Here's how the part is built. I have some questions about the finished solid (model axes, mm). A direction names the side the tool comes from. Round coordinates to 2 decimals unless told otherwise and drop trailing zeros. One line per item, written item: value. Start each with the question number.
```python
from build123d import *

# Parameters (mm, degrees)
BOSS_EXTRUDE1_DEPTH = 5
SKETCH4_W           = 22
SKETCH4_H           = 25.575781223
CUT_EXTRUDE1_DEPTH  = 5
CUT_EXTRUDE2_DEPTH  = 5
SKETCH10_W          = 47.253020793
SKETCH10_H          = 79.148030785
CUT_EXTRUDE3_DEPTH  = 5
MIRROR8_DEPTH       = 5
SKETCH11_R          = 10.33
CUT_EXTRUDE4_DEPTH  = 5
FILLET5_R           = 2


# Read off the part's stored shape, not the designer's step: Mirror8
with BuildPart() as part:
    # Sketch3 → Boss-Extrude1 (new body)
    with BuildSketch(Plane(origin=(0, 0, 0), x_dir=(1, 0, 0), z_dir=(0, 1, 0))):
        Polygon((35, 0), (24.748737342, 24.748737342), (0, 35), (-24.748737342, 24.748737342), (-35, 0), (-24.748737342, -24.748737342), (0, -35), (24.748737342, -24.748737342), align=None)
    extrude(amount=BOSS_EXTRUDE1_DEPTH)

    # Sketch4 → Cut-Extrude1 (cut)
    with BuildSketch(Plane(origin=(0, 5, 0), x_dir=(1, 0, 0), z_dir=(0, 1, 0))):
        with Locations((-11.044164743, -6.541737694)):
            Rectangle(SKETCH4_W, SKETCH4_H)
    extrude(amount=-CUT_EXTRUDE1_DEPTH, mode=Mode.SUBTRACT)

    # Sketch4<6> → Cut-Extrude2 (cut)
    with BuildSketch(Plane(origin=(0, 5, 0), x_dir=(1, 0, 0), z_dir=(0, 1, 0))):
        with BuildLine():
            ThreePointArc((-22.044164743, 6.246152918), (-11.044164743, 10.694704781), (-0.044164743, 6.246152918))
            Line((-0.044164743, 6.246152918), (-22.044164743, 6.246152918))
        make_face()
        with BuildLine():
            Line((-22.044164743, -19.329628305), (-0.044164743, -19.329628305))
            ThreePointArc((-0.044164743, -19.329628305), (-11.044164743, -23.778180168), (-22.044164743, -19.329628305))
        make_face()
    extrude(amount=-CUT_EXTRUDE2_DEPTH, mode=Mode.SUBTRACT)

    # Sketch10 → Cut-Extrude3 (cut)
    with BuildSketch(Plane(origin=(0, 5, 0), x_dir=(1, 0, 0), z_dir=(0, 1, 0))):
        with Locations((23.626510397, -1.493894903)):
            Rectangle(SKETCH10_W, SKETCH10_H)
    extrude(amount=-CUT_EXTRUDE3_DEPTH, mode=Mode.SUBTRACT)

    # Mirror8 outline → Mirror8 (add)
    with BuildSketch(Plane(origin=(0, 0, 0), x_dir=(1, 0, 0), z_dir=(0, 1, 0))):
        Polygon((24.748737342, 24.748737342), (0, 35), (0, -35), (24.748737342, -24.748737342), (35, 0), align=None)
        with BuildLine():
            ThreePointArc((0.044164743, 6.246152918), (11.044164743, 10.694704781), (22.044164743, 6.246152918))
            Line((22.044164743, 6.246152918), (22.044164743, -19.329628305))
            ThreePointArc((22.044164743, -19.329628305), (11.044164743, -23.778180168), (0.044164743, -19.329628305))
            Line((0.044164743, -19.329628305), (0.044164743, 6.246152918))
        make_face(mode=Mode.SUBTRACT)
    extrude(amount=MIRROR8_DEPTH)

    # Sketch11 → Cut-Extrude4 (cut)
    with BuildSketch(Plane(origin=(0, 5, 0), x_dir=(1, 0, 0), z_dir=(0, 1, 0))):
        with Locations(Location((0, 18.670604022, 0), (0, 0, 270))):
            Circle(SKETCH11_R)
    extrude(amount=-CUT_EXTRUDE4_DEPTH, mode=Mode.SUBTRACT)

    # Fillet5
    fillet5_edges = [part.edges().sort_by_distance(p)[0] for p in [
        (-12.374368671, 5, -29.874368671),
        (-29.874368671, 5, -12.374368671),
        (-29.874368671, 5, 12.374368671),
        (-12.374368671, 5, 29.874368671),
        (12.374368671, 5, -29.874368671),
        (29.874368671, 5, -12.374368671),
        (29.874368671, 5, 12.374368671),
        (12.374368671, 0, -29.874368671),
        (29.874368671, 0, -12.374368671),
        (29.874368671, 0, 12.374368671),
        (12.374368671, 0, 29.874368671),
        (12.374368671, 5, 29.874368671),
        (-12.374368671, 0, 29.874368671),
        (-29.874368671, 0, 12.374368671),
        (-29.874368671, 0, -12.374368671),
        (-12.374368671, 0, -29.874368671),
    ]]
    fillet(fillet5_edges, radius=FILLET5_R)


solid = part.part
```
Q1. Will these pins go through, and if not, where does the flat tip stop? P1, Ø1.5, axis at y = 1.5, z = 6.5, coming from the +X side; P2, Ø1.5, axis at y = 2, z = 1.5, coming from the -X side; P3, Ø1, axis at x = 13, y = 3.5, coming from the +Z side.
Q2. I want a section at A-A on z = 8.5. State how many separate pieces and enclosed holes the cut face has, plus the area to 3 significant figures.
Q3. If we mould it in two halves opening along X, with no side actions, what happens to faces 3 (the cylindrical face through (10.874, 2.465, -10.694)), 4 (the cylindrical face through (-29.39, 4.43, -11.97)), 5 (the flat face through (29.946, 2.493, -12.201))? For each: released by +X, released by -X, zero draft, split by the parting line, or undercut.
Q4. Which directions (+Z, -Z, +X, -X, +Y, -Y) give clear straight access to the entire face, cutting with the end or side of a thin tool? Please do faces 1 (the flat face through (12.55, 2.49, -29.8)), 2 (the cylindrical face through (-10.874, 2.535, 23.777)).
Q5. If I drill on line 1 along X through (y, z) = (2.8, -7); line 2 along Z through (x, y) = (-8.5, 2.45); line 3 along X through (y, z) = (1.4, -8), over which ranges is the centre line in solid material (lowest first)?
Answers below:
1. P1: stops at x = 32.58
1. P2: stops at x = -34.69
1. P3: stops at z = 29.78
2. separate pieces: 3
2. enclosed holes: 0
2. area: 91.1 mm^2
3. face 3: undercut
3. face 4: released by -X
3. face 5: released by +X
4. face 1: -Z, +X, +Y, -Y
4. face 2: +Y, -Y
5. line 1: x = -32.1 to -21.21, -0.88 to 0.88, 21.21 to 32.1
5. line 2: z = -31.48 to -24.54, -12.8 to -10.49, 23.57 to 31.48
5. line 3: x = -31.59 to -19.88, -2.21 to 2.21, 19.88 to 31.59
